```python
from build123d import *

# Parameters (mm, degrees)
BOX_W             = 14.25
BOX_H             = 30
BOX_DEPTH         = 20
CYLINDER002_R     = 21.15
CYLINDER002_DEPTH = 30
CYLINDER001_R     = 22.5
CYLINDER001_DEPTH = 20
FILLET_R          = 1
FILLET001_R       = 1
CYLINDER_R        = 25.5
CYLINDER_DEPTH    = 2.5


with BuildPart() as cube:
    # Box → Box (new body)
    with BuildSketch(Plane(origin=(-7.125, 0, 2.5), x_dir=(1, 0, 0), z_dir=(0, 0, 1))):
        with Locations((7.125, 15)):
            Rectangle(BOX_W, BOX_H)
    extrude(amount=BOX_DEPTH)


with BuildPart() as cylinder002:
    # Cylinder002 → Cylinder002 (new body)
    with BuildSketch(Plane.XY.offset(2.5)):
        Circle(CYLINDER002_R)
    extrude(amount=CYLINDER002_DEPTH)


with BuildPart() as fillet001:
    # Cylinder001 → Cylinder001 (new body)
    with BuildSketch(Plane.XY):
        Circle(CYLINDER001_R)
    extrude(amount=CYLINDER001_DEPTH)

    # Cut: cut Cylinder002
    add(cylinder002.part, mode=Mode.SUBTRACT)

    # Cut001: cut Cube
    add(cube.part, mode=Mode.SUBTRACT)

    # Fillet
    fillet_edges = [fillet001.edges().sort_by_distance(p)[0] for p in [
        (-12.178439, -17.291851, 20),
        (17.291851, 12.178439, 20),
    ]]
    fillet(fillet_edges, radius=FILLET_R)

    # Fillet001
    fillet001_edges = [fillet001.edges().sort_by_distance(p)[0] for p in [
        (-7.125, 21.157422, 20),
        (7.125, 21.157422, 20),
        (-7.125, 20.235006, 19.716842),
        (7.125, 20.235006, 19.716842),
    ]]
    fillet(fillet001_edges, radius=FILLET001_R)


with BuildPart() as viewfinder_cap:
    # Cylinder → Cylinder (new body)
    with BuildSketch(Plane.XY):
        Circle(CYLINDER_R)
    extrude(amount=CYLINDER_DEPTH)

    # Fusion: union Fillet001
    add(fillet001.part)


solid = viewfinder_cap.part
```
Build history of the part. All positions in model axes, mm. A direction names the side the tool comes from. Coordinates: 2 decimals unless noted, no trailing zeros. Order: outer loops, then holes, each group sorted by start corner. A loop starts at its lowest first (then second) coordinate and runs counter-clockwise, first axis right, second up.
Item 1: Saw through at A-A on z = 7.25. List the corners of the cut face in (x, y) (3 decimals), then the cut area to 3 significant figures.
Filled in:
outline: (-7.758, 19.676) arc R1 ccw to (-7.125, 20.606) - (-7.125, 21.342) arc R22.5 ccw (long way) to (7.125, 21.342) - (7.125, 20.606) arc R1 ccw to (7.758, 19.676) arc R21.15 cw (long way) to start
area: 165 mm2
Item 2: Saw through at C-C on y = 0. List the corners of the cut face in (x, z).
Filled in:
outline: (-25.5, 0) - (25.5, 0) - (25.5, 2.5) - (22.5, 2.5) - (22.5, 20) - (22.15, 20) arc R1 ccw to (21.15, 19) - (21.15, 2.5) - (-21.15, 2.5) - (-21.15, 19) arc R1 ccw to (-22.15, 20) - (-22.5, 20) - (-22.5, 2.5) - (-25.5, 2.5) - close
Item 3: Drill centre lines: L1, parallel to X at y = 0, z = 12.25; L2, parallel to Z at x = 13, y = -1.5; L3, parallel to Y at x = 0, z = 15. Where is each one in solid material? Low to high.
Filled in:
L1: x = -22.5 to -21.15, 21.15 to 22.5
L2: z = 0 to 2.5
L3: y = -22.5 to -21.15
Item 4: Saw through at B-B on x = 0. List the corners of the cut face in (y, z), then the cut area to 3 significant figures.
Filled in:
outline: (-25.5, 0) - (25.5, 0) - (25.5, 2.5) - (-21.15, 2.5) - (-21.15, 19) arc R1 ccw to (-22.15, 20) - (-22.5, 20) - (-22.5, 2.5) - (-25.5, 2.5) - close
area: 151 mm2
Item 5: Tool access for faces 1 (the flat face through (0, 0, 2.5)), 2 (the flat face through (0, 0, 0)): list every direction of +Z, -Z, +X, -X, +Y, -Y with a clear straight run to the whole face (end or side of a thin tool).
Filled in:
face 1: +Z
face 2: -Z, +X, -X, +Y, -Y
Item 6: Drop flat-ended pins along their axis: pin 1 Ø12 at (y, z) = (15.5, 4.5) entering from -X; pin 2 Ø1 at (x, z) = (13, 11) entering from -Y; pin 3 Ø10 at (y, z) = (13.5, 9.5) entering from -X. Give the stop position or say it passes through.
Filled in:
pin 1: stops at x = -23.52
pin 2: stops at y = -18.71
pin 3: stops at x = -20.83
